Input: part model. Units: mm. Frame: model coordinates. Face numbers are marked on the shaded views. A direction names the side the tool comes from. Round coordinates to 2 decimals unless told otherwise and drop trailing zeros. Loops run counter-clockwise (first coordinate to the right, second up) from the corner with the lowest first, then second, coordinate; pieces in that order, holes last.
(1) First-contact query: pin 1 Ø10 at (x, z) = (23.5, 27) entering from +Y; pin 2 Ø4 at (x, y) = (21.5, 28.5) entering from +Z. Flat tips, straight axial feed; report the tip coordinate or a pass-through.
(2) Line query: line 1 (Y direction, x = 29, z = 37.5); line 2 (X direction, y = 16.5, z = 23); line 3 (X direction, y = 60, z = 2). Output: solid intervals per line, ascending.
(3) Cut plane B-B, the plane y = 8. Output: boundary loops of the cut face in (x, z).
(4) Access query for the marked faces 1, 2 and 3. Directions: +Z, -Z, +X, -X, +Y, -Y. A direction counts if a zero-diameter tool reaches every point of the face in a straight line with its end or side. Return the directions, or none.
(5) Cut plane D-D, the plane x = 8. Output: boundary loops of the cut face in (y, z).
(6) Cut plane A-A, the plane y = 34.5. Output: boundary loops of the cut face in (x, z), and give its area (3 significant figures).
(7) Draft query along Y for the marked faces 4, 5 and 6. Return one class per face: released by +Y, released by -Y, zero draft, split by the parting line, or undercut.
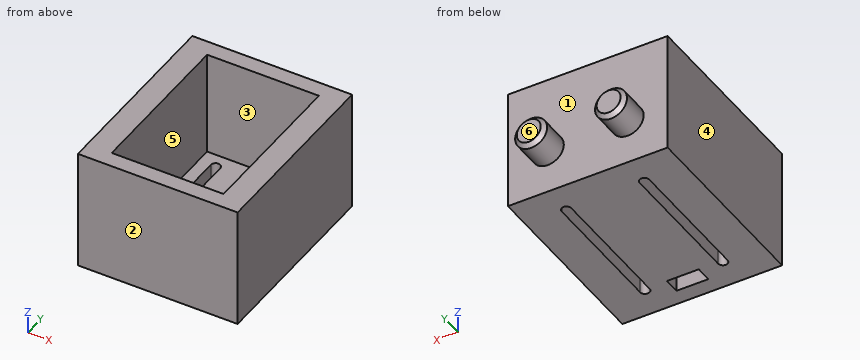
from build123d import *

# Parameters (mm, degrees)
SKETCH2_W               = 63.5
SKETCH2_H               = 76.2
BOSS_EXTRUDE1_DEPTH     = 48.26
SKETCH3_W               = 44.45
SKETCH3_H               = 63.5
CUT_EXTRUDE1_DEPTH      = 41.91
CUT_EXTRUDE2_DEPTH      = 108.680722973
CUT_EXTRUDE2_DEPTH_BACK = 108.680722973
SKETCH4_W               = 12.7
SKETCH4_H               = 6.35
SKETCH5_R               = 6.35
BOSS_EXTRUDE2_DEPTH     = 12.7
CHAMFER1_SIZE           = 1.5875


with BuildPart() as part:
    # Sketch2 → Boss-Extrude1 (new body)
    with BuildSketch(Plane.XY):
        with Locations((31.75, 38.1)):
            Rectangle(SKETCH2_W, SKETCH2_H)
    extrude(amount=BOSS_EXTRUDE1_DEPTH)

    # Sketch3 → Cut-Extrude1 (cut)
    with BuildSketch(Plane.XY.offset(48.26)):
        with Locations((31.877, 38.1)):
            Rectangle(SKETCH3_W, SKETCH3_H)
    extrude(amount=-CUT_EXTRUDE1_DEPTH, mode=Mode.SUBTRACT)

    # Sketch4 → Cut-Extrude2 (cut, two sides: drawn at the far end of the back side and taken through both)
    with BuildSketch(Plane.XY.offset(6.35).offset(-CUT_EXTRUDE2_DEPTH_BACK)):
        with Locations((31.877, 9.525)):
            Rectangle(SKETCH4_W, SKETCH4_H)
        with BuildLine():
            Line((18.2626, 64.1985), (18.2626, 12.0015))
            ThreePointArc((18.2626, 12.0015), (16.383, 10.1219), (14.5034, 12.0015))
            Line((14.5034, 12.0015), (14.5034, 64.1985))
            ThreePointArc((14.5034, 64.1985), (16.383, 66.0781), (18.2626, 64.1985))
        make_face()
        with BuildLine():
            Line((49.2506, 64.1985), (49.2506, 12.0015))
            ThreePointArc((49.2506, 12.0015), (47.371, 10.1219), (45.4914, 12.0015))
            Line((45.4914, 12.0015), (45.4914, 64.1985))
            ThreePointArc((45.4914, 64.1985), (47.371, 66.0781), (49.2506, 64.1985))
        make_face()
    extrude(amount=CUT_EXTRUDE2_DEPTH + CUT_EXTRUDE2_DEPTH_BACK, mode=Mode.SUBTRACT)

    # Sketch5 → Boss-Extrude2 (add)
    with BuildSketch(Plane(origin=(0, 76.2, 0), x_dir=(1, 0, 0), z_dir=(0, 1, 0))):
        with Locations(Location((15.875, -17.78, 0), (0, 0, 90))):
            Circle(SKETCH5_R)
        with Locations(Location((47.625, -17.78, 0), (0, 0, 90))):
            Circle(SKETCH5_R)
    extrude(amount=BOSS_EXTRUDE2_DEPTH)

    # Chamfer1
    chamfer1_edges = [part.edges().sort_by_distance(p)[0] for p in [
        (15.875, 88.9, 24.13),
        (47.625, 88.9, 24.13),
    ]]
    chamfer(chamfer1_edges, length=CHAMFER1_SIZE)


solid = part.part
Reported:
1. pin 1: stops at y = 76.2
1. pin 2: stops at z = 6.35
2. line 1: y = 0 to 6.35, 69.85 to 76.2
2. line 2: x = 0 to 9.65, 54.1 to 63.5
2. line 3: x = 0 to 14.5, 18.26 to 45.49, 49.25 to 63.5
3. outline: (0, 0) - (25.53, 0) - (25.53, 6.35) - (9.65, 6.35) - (9.65, 48.26) - (0, 48.26) - close; (38.23, 0) - (63.5, 0) - (63.5, 48.26) - (54.1, 48.26) - (54.1, 6.35) - (38.23, 6.35) - close
4. face 1: +Y
4. face 2: +Z, -Z, +X, -X, -Y
4. face 3: +Z
5. outline: (0, 0) - (76.2, 0) - (76.2, 48.26) - (0, 48.26) - close
6. outline: (0, 0) - (14.5, 0) - (14.5, 6.35) - (9.65, 6.35) - (9.65, 48.26) - (0, 48.26) - close; (18.26, 0) - (45.49, 0) - (45.49, 6.35) - (18.26, 6.35) - close; (49.25, 0) - (63.5, 0) - (63.5, 48.26) - (54.1, 48.26) - (54.1, 6.35) - (49.25, 6.35) - close
6. area: 1,150 mm2
7. face 4: zero draft
7. face 5: undercut
7. face 6: released by +Y
